from build123d import *

# Parameters (mm, degrees)
BOSS_EXTRUDE1_DEPTH      = 10
BOSS_EXTRUDE1_DEPTH_BACK = 10
SKETCH3_W                = 20
SKETCH3_H                = 62
FILLET1_R                = 3
SKETCH4_R                = 2.75
CUT_EXTRUDE1_DEPTH       = 64.592452382
CHAMFER1_SIZE            = 1.5
CHAMFER2_SIZE            = 3


with BuildPart() as part:
    # Sketch3 → Boss-Extrude1 (new, two sides: drawn at the far end of the back side and taken through both)
    with BuildSketch(Plane(origin=(0, 0, 0), x_dir=(0, 0, -1), z_dir=(1, 0, 0)).offset(-BOSS_EXTRUDE1_DEPTH_BACK)):
        with Locations((0, 31)):
            Rectangle(SKETCH3_W, SKETCH3_H)
    extrude(amount=BOSS_EXTRUDE1_DEPTH + BOSS_EXTRUDE1_DEPTH_BACK)

    # Fillet1
    fillet1_edges = [part.edges().sort_by_distance(p)[0] for p in [
        (10, 31, 10),
        (-10, 31, 10),
    ]]
    fillet(fillet1_edges, radius=FILLET1_R)

    # Sketch4 → Cut-Extrude1 (cut, through all)
    with BuildSketch(Plane(origin=(0, 62, 0), x_dir=(1, 0, 0), z_dir=(0, 1, 0))):
        Circle(SKETCH4_R)
        with BuildLine():
            ThreePointArc((1.944543648, -1.944543648), (0, -2.75), (-1.944543648, -1.944543648))
            Line((-1.944543648, -1.944543648), (0, -3.889087297))
            Line((0, -3.889087297), (1.944543648, -1.944543648))
        make_face()
    extrude(amount=-CUT_EXTRUDE1_DEPTH, mode=Mode.SUBTRACT)

    # Chamfer1
    chamfer1_edges = [part.edges().sort_by_distance(p)[0] for p in [
        (0, 62, -2.75),
        (-0.972271824, 62, 2.916815472),
        (0.972271824, 62, 2.916815472),
    ]]
    chamfer(chamfer1_edges, length=CHAMFER1_SIZE)

    # Chamfer2
    chamfer2_edges = [part.edges().sort_by_distance(p)[0] for p in [
        (-10, 31, -10),
        (10, 31, -10),
    ]]
    chamfer(chamfer2_edges, length=CHAMFER2_SIZE)


solid = part.part
Read the model definition and answer for the solid it produces. Units are mm, in the model's axes. A direction names the side the tool comes from. Give positions to 0.01 mm unless a question says otherwise; leave off trailing zeros. Write each loop counter-clockwise with the first axis right and the second up, starting at its lowest first coordinate (ties: lowest second). Pieces come first, ordered by that corner, then holes. Notation, with made-up numbers: (5.5, 6.5) - (11.5, 6.5) arc R19 ccw to (11.5, 39.5) - close; hole circle Ø8 at (59, 20.5). An arc over 180 degrees is marked (long way). Answer in a Markdown table with one row per item. Add a question column.
Item 1: Find the intervals of material crossed by L1, parallel to X at y = 30, z = 0; L2, parallel to Z at x = -2, y = 15; L3, parallel to Z at x = 0.25, y = 47, in increasing order.
Item 2: Section B-B, the plane y = 11 is taken. Write down the section's boundary in (x, z).
Item 3: Determine the mould class of faces 1 (the face through (-9.1, 31.43, 9.14)), 2 (the face through (0.96, 30.67, 2.93)), 3 (the face through (-10, 31, 0)) for opening direction Z: pulls with the +Z half, pulls with the -Z half, needs draft (parallel to the pull), parting line crosses it, or undercut.
Item 4: Section A-A, the plane z = 0 is taken. Write down the section's boundary in (x, y).
Item 5: A tool of negligible diameter and unlimited length cuts with its end or side. For faces 4 (the face through (1.278, 61.24, 3.657)), 5 (the face through (0, 31, -10)), 6 (the face through (-0.99, 30.67, 2.9)), from which of +Z, -Z, +X, -X, +Y, -Y can it reach the whole face along a straight path? Write none if from no direction.
Item 6: Section C-C, the plane x = 8 is taken. Write down the section's boundary in (y, z).
Recorded:
| question | item | result |
|---|---|---|
| 1 | L1 | x = -10 to -2.75, 2.75 to 10 |
| 1 | L2 | z = -10 to -1.89, 1.89 to 10 |
| 1 | L3 | z = -10 to -2.74, 3.64 to 10 |
| 2 | outline | (-10, -7) - (-7, -10) - (7, -10) - (10, -7) - (10, 7) arc R3 ccw to (7, 10) - (-7, 10) arc R3 ccw to (-10, 7) - close; hole (-1.94, 1.94) arc R2.75 ccw (long way) to (1.94, 1.94) - (0, 3.89) - close |
| 3 | face 1 | pulls with the +Z half |
| 3 | face 2 | undercut |
| 3 | face 3 | needs draft |
| 4 | outline | (-10, 0) - (-2.75, 0) - (-2.75, 60.5) - (-4.25, 62) - (-10, 62) - close; (2.75, 0) - (10, 0) - (10, 62) - (4.25, 62) - (2.75, 60.5) - close |
| 5 | face 4 | +Y |
| 5 | face 5 | -Z, +X, -X, +Y, -Y |
| 5 | face 6 | +Y, -Y |
| 6 | outline | (0, -9) - (62, -9) - (62, 9.83) - (0, 9.83) - close |
